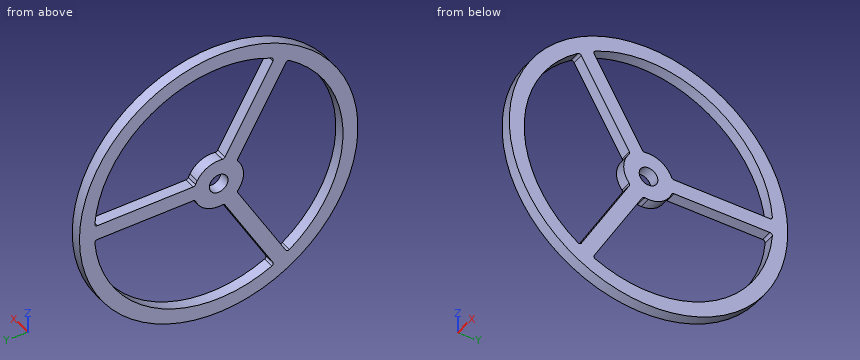
Autodesk Inventor part; units mm, degrees
ref_plane "YZ Plane" through (0, 0, 0) normal (1, 0, 0) x (0, 1, 0)
ref_plane "XZ Plane" through (0, 0, 0) normal (0, 1, 0) x (-1, 0, 0)
ref_plane "XY Plane" through (0, 0, 0) normal (0, 0, 1) x (1, 0, 0)
sketch "Sketch1" plane through (0, 0, 0) normal (1, 0, 0) x (0, 1, 0)
  circle A0 centre (0, 0) radius 7.5
  circle A1 centre (0, 0) radius 111.9
  dimension "D_eje" = 15
  dimension "d1" = 223.8
extrude "Extrusion1" add sketch "Sketch1" along normal blind 9
sketch "Sketch2" plane through (9, 0, 0) normal (1, 0, 0) x (0, 0, -1)
  line L0 (6, 19.0264) -> (6, 99.7197)
  line L1 (0, -188.1875) -> (0, 173.8632) construction
  arc A0 (0, 19.95) -> (-13.4773, 14.7093) centre (0, 0) ccw construction
  circle A1 centre (0, 0) radius 7.5 construction
  arc A2 (0, 99.9) -> (86.5159, -49.95) centre (0, 0) ccw construction
  line L2 (181.1282, 0) -> (-189.3983, 0) construction
  arc A3 (6, 19.0264) -> (0, 19.95) centre (0, 0) ccw construction
  arc A4 (-19.95, 0) -> (0, -19.95) centre (0, 0) ccw construction
  arc A5 (0, -19.95) -> (17.2772, -9.975) centre (0, 0) ccw construction
  arc A6 (19.95, 0) -> (6, 19.0264) centre (0, 0) ccw
  line L3 (0, 0) -> (86.5159, -49.95) construction
  line L4 (19.4773, -4.317) -> (89.3598, -44.6637)
  arc A7 (-13.4773, 14.7093) -> (-19.95, 0) centre (0, 0) ccw construction
  arc A8 (19.4773, -4.317) -> (19.95, 0) centre (0, 0) ccw
  arc A9 (17.2772, -9.975) -> (19.4773, -4.317) centre (0, 0) ccw construction
  arc A10 (6, 99.7197) -> (0, 99.9) centre (0, 0) ccw construction
  arc A11 (86.5159, -49.95) -> (89.3598, -44.6637) centre (0, 0) ccw construction
  arc A12 (89.3598, -44.6637) -> (6, 99.7197) centre (0, 0) ccw
  line L5 (-19.4773, -4.317) -> (-89.3598, -44.6637)
  arc A13 (-6, 99.7197) -> (-89.3598, -44.6637) centre (0, 0) ccw
  line L6 (-6, 19.0264) -> (-6, 99.7197)
  arc A14 (-9.975, 17.2772) -> (-19.4773, -4.317) centre (0, 0) ccw
  line L7 (13.4773, -14.7093) -> (83.3598, -55.056)
  arc A15 (-83.3598, -55.056) -> (83.3598, -55.056) centre (0, 0) ccw
  line L8 (-13.4773, -14.7093) -> (-83.3598, -55.056)
  arc A16 (-9.975, -17.2772) -> (13.4773, -14.7093) centre (0, 0) ccw
  point P0 (-6, -19.0264)
  point P1 (19.4773, 4.317)
  dimension "d4" = 6
  dimension "d7" = 39.9
  dimension "d8" = 199.8
  dimension "d10" = 120
  dimension "d11" = 6
  dimension "d14" = 360
extrude "Extrusion2" cut sketch "Sketch2" against normal blind 9
pattern_circular "Circular Pattern1" count 3 over 360 about axis through (-10, 0, 0) along (1, 0, 0) of "Extrusion2"
fillet "Fillet1" radius 2 12 edges at (4.5, -14.7093, -13.4773) (4.5, -14.7093, 13.4773) (4.5, -55.056, 83.3598) (4.5, -55.056, -83.3598) (4.5, -44.6637, -89.3598) (4.5, 99.7197, -6) (4.5, -4.317, -19.4773) (4.5, 19.0264, -6) (4.5, 19.0264, 6) (4.5, -4.317, 19.4773) (4.5, 99.7197, 6) (4.5, -44.6637, 89.3598)
properties part number "Rueda_triciclo" material "Aluminum 6061"
Can you work these out from the model? Positions are in its coordinate system, mm. Coordinates: 2 decimals unless noted, no trailing zeros. Write each loop counter-clockwise with the first axis right and the second up, starting at its lowest first coordinate (ties: lowest second). Pieces come first, ordered by that corner, then holes.
Q1. Imagine slicing it at A-A, the plane z = 0. List the corners of the cut face in (x, y) for me, plus the area to 3 significant figures.
Results found:
outline: (0, -111.9) - (9, -111.9) - (9, -99.9) - (0, -99.9) - close; (0, -19.95) - (9, -19.95) - (9, -7.5) - (0, -7.5) - close; (0, 7.5) - (9, 7.5) - (9, 111.9) - (0, 111.9) - close
area: 1,160 mm2
Q2. Imagine slicing it at C-C, the plane y = 84. List the corners of the cut face in (x, z) for me.
Results found:
outline: (0, -73.93) - (9, -73.93) - (9, -54.07) - (0, -54.07) - close; (0, -6) - (9, -6) - (9, 6) - (0, 6) - close; (0, 54.07) - (9, 54.07) - (9, 73.93) - (0, 73.93) - close
Q3. For P1, Ø4.5, axis at x = 2.5, y = 69.5, coming from the -Z side; P2, Ø4, axis at x = 3, z = 27.5, coming from the -Y side; P3, Ø5, axis at x = 3, y = -70.5, coming from the -Z side, each with a flat end and sliding along its axis, tell me the tip position at first contact or that it passes through.
Results found:
P1: stops at z = -89.44
P2: stops at y = -108.96
P3: stops at z = -88.87
Q4. Imagine slicing it at B-B, the plane y = -80.5. List the corners of the cut face in (x, z) for me, plus the area to 3 significant figures.
Results found:
outline: (0, -77.73) - (9, -77.73) - (9, -59.16) - (0, -59.16) - close; (0, 59.16) - (9, 59.16) - (9, 77.73) - (0, 77.73) - close
area: 334 mm2
Q5. Imagine slicing it at D-D, the plane y = -39.5. List the corners of the cut face in (x, z) for me, plus the area to 3 significant figures.
Results found:
outline: (0, -104.7) - (9, -104.7) - (9, -91.76) - (0, -91.76) - close; (0, -80.42) - (9, -80.42) - (9, -56.42) - (0, -56.42) - close; (0, 56.42) - (9, 56.42) - (9, 80.42) - (0, 80.42) - close; (0, 91.76) - (9, 91.76) - (9, 104.7) - (0, 104.7) - close
area: 665 mm2
Q6. Please list where these lines run through material, in increasing order: L1, parallel to Z at x = 5, y = 0; L2, parallel to Z at x = 5.75, y = -15; L3, parallel to Z at x = 6.75, y = 24.
Results found:
L1: z = -111.9 to -99.9, -19.95 to -7.5, 7.5 to 19.95, 99.9 to 111.9
L2: z = -110.89 to -98.77, -37.98 to 37.98, 98.77 to 110.89
L3: z = -109.3 to -96.97, -6 to 6, 96.97 to 109.3
